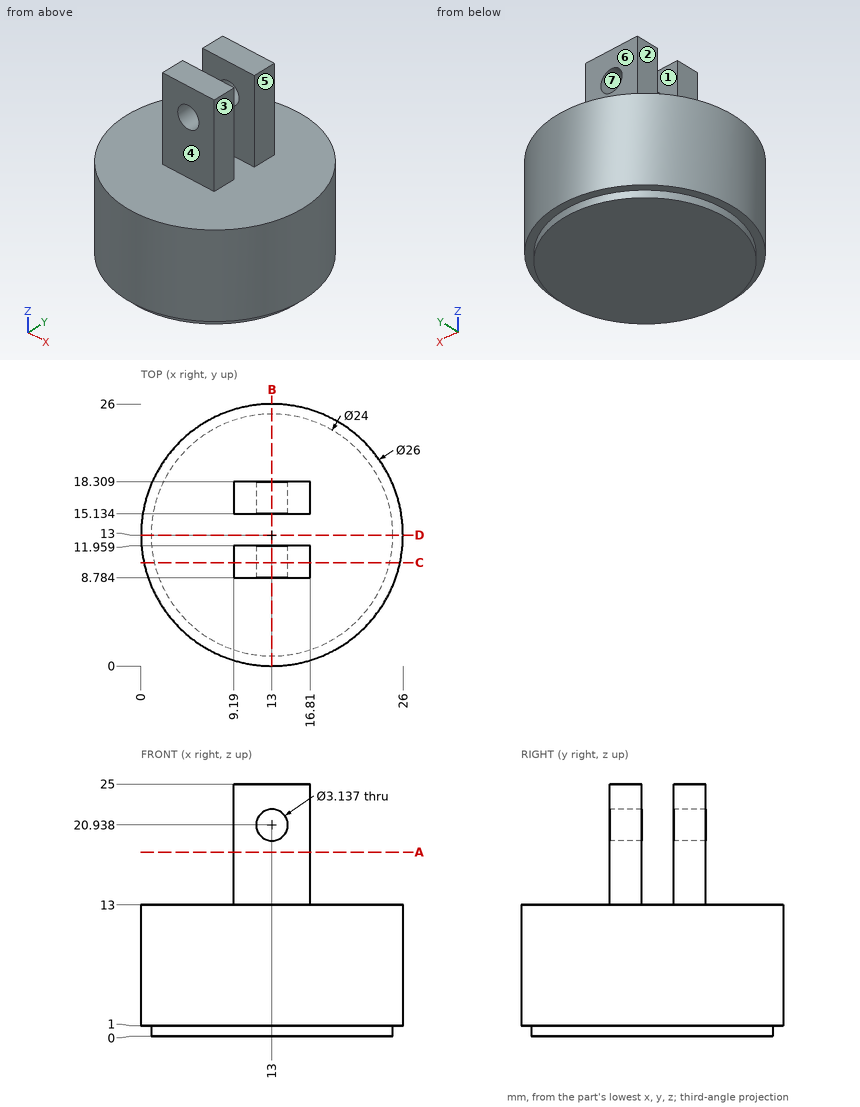
Design review of the part shown in the three views and the two pictorial views. Dimensions are in mm from the part's minimum x, y and z. A direction names the side the tool comes from. Coordinates: 2 decimals unless noted, no trailing zeros. Loops run counter-clockwise (first coordinate to the right, second up) from the corner with the lowest first, then second, coordinate; pieces in that order, holes last.
Q1. For pin 1 (1 mm diameter, centred on y = 10, z = 19.5, fed in from -X); pin 2 (1.9 mm diameter, centred on x = 13, z = 20.94, fed in from -Y); pin 3 (3.5 mm diameter, centred on x = 13, z = 20.94, fed in from -Y); pin 4 (1.5 mm diameter, centred on y = 22.5, z = 10, fed in from -X) (1 decimal), all flat-tipped, find the tip position at first contact; note any pin that passes through.
Reported:
pin 1: stops at x = 9.19
pin 2: passes through
pin 3: stops at y = 8.78
pin 4: stops at x = 3.4
Q2. We need section D-D on y = 13. State the section outline as (x, z) points.
Reported:
outline: (0, 1) - (1, 1) - (1, 0) - (25, 0) - (25, 1) - (26, 1) - (26, 13) - (0, 13) - close
Q3. We need section B-B on x = 13. State the section outline as (y, z) points (1 decimal), and give its area (3 significant figures).
Reported:
outline: (0, 1) - (1, 1) - (1, 0) - (25, 0) - (25, 1) - (26, 1) - (26, 13) - (18.3, 13) - (18.3, 19.4) - (15.1, 19.4) - (15.1, 13) - (12, 13) - (12, 19.4) - (8.8, 19.4) - (8.8, 13) - (0, 13) - close; (8.8, 22.5) - (12, 22.5) - (12, 25) - (8.8, 25) - close; (15.1, 22.5) - (18.3, 22.5) - (18.3, 25) - (15.1, 25) - close
area: 392 mm2
Q4. To check wall thickness, follow line 1 (Z direction, x = 13, y = 11.15) (1 decimal); line 2 (Y direction, x = 10.5, z = 17); line 3 (Z direction, x = 17.25, y = 1). State the ranges of each line that lie inside material, in increasing order.
Reported:
line 1: z = 0 to 19.4, 22.5 to 25
line 2: y = 8.78 to 11.96, 15.13 to 18.31
line 3: z = 1 to 13
Q5. Tool access review of the marked faces 1, 2, 3 and 4: name each direction out of +Z, -Z, +X, -X, +Y, -Y from which nothing blocks a thin tool from reaching the whole face with its end or side.
Reported:
face 1: +Z, +X, -X
face 2: +Z, -X, +Y, -Y
face 3: +Z, +X, +Y, -Y
face 4: +Z, +X, -X, -Y
Q6. We need section A-A on z = 18.25. State the section outline as (x, y) points.
Reported:
outline: (9.19, 8.78) - (16.81, 8.78) - (16.81, 11.96) - (9.19, 11.96) - close; (9.19, 15.13) - (16.81, 15.13) - (16.81, 18.31) - (9.19, 18.31) - close
Q7. The part is to be moulded in two halves that separate along X. For the marked faces 5, 6 and 7, say which applies: +X half, -X half, draft (parallel to the pull), parting line (faces both ways), or undercut.
Reported:
face 5: +X half
face 6: draft
face 7: undercut
Q8. We need section C-C on y = 10.25. State the section outline as (x, z) points (1 decimal), and give its area (3 significant figures).
Reported:
outline: (0.3, 1) - (1.3, 1) - (1.3, 0) - (24.7, 0) - (24.7, 1) - (25.7, 1) - (25.7, 13) - (16.8, 13) - (16.8, 25) - (9.2, 25) - (9.2, 13) - (0.3, 13) - close; hole circle Ø3.1 at (13, 20.9)
area: 412 mm2
